Design review of the part shown in the three views and the two pictorial views. Dimensions are in mm from the part's minimum x, y and z. A direction names the side the tool comes from. Coordinates: 2 decimals unless noted, no trailing zeros. Loops run counter-clockwise (first coordinate to the right, second up) from the corner with the lowest first, then second, coordinate; pieces in that order, holes last. Notation, with made-up numbers: (22, -21) -> (78, -21) arc R20 ccw to (78, 16) -> close; hole circle Ø6 at (47.5, -15.5). An arc over 180 degrees is marked (long way). One line per item, written item: value. Start each with the question number.
1. Add section C-C on y = 33.5. Write out the cut boundary in (x, z), plus the area to 3 significant figures.
2. Add section A-A on y = 17.5. Write out the cut boundary in (x, z).
3. For probe 1 along X at (y, z) = (15, 6); probe 2 along Y at (x, z) = (80.2, 2.5); probe 3 along X at (y, z) = (46, 18.25), list the stretches that pass through material, from the lowest coordinate up.
4. Add section D-D on x = 16. Write out the cut boundary in (y, z).
5. Insertion check: pin 1 (2.5 mm diameter, centred on x = 80, z = 10, fed in from +Y); pin 2 (1.5 mm diameter, centred on x = 80.5, z = 1.5, fed in from -Y); pin 3 (4 mm diameter, centred on x = 72.5, z = 13.5, fed in from +Y). Each pin has a flat end and moves straight along its axis. Give the tip position at first contact, or say it passes through.
6. Machinability: for the marked faces 1, 2 and 3, which of the approach directions +Z, -Z, +X, -X, +Y, -Y give a long, thin tool a straight path to every point of the face, cutting with its end or side? Answer none if there is none.
7. Add section B-B on z = 2.5. Write out the cut boundary in (x, y).
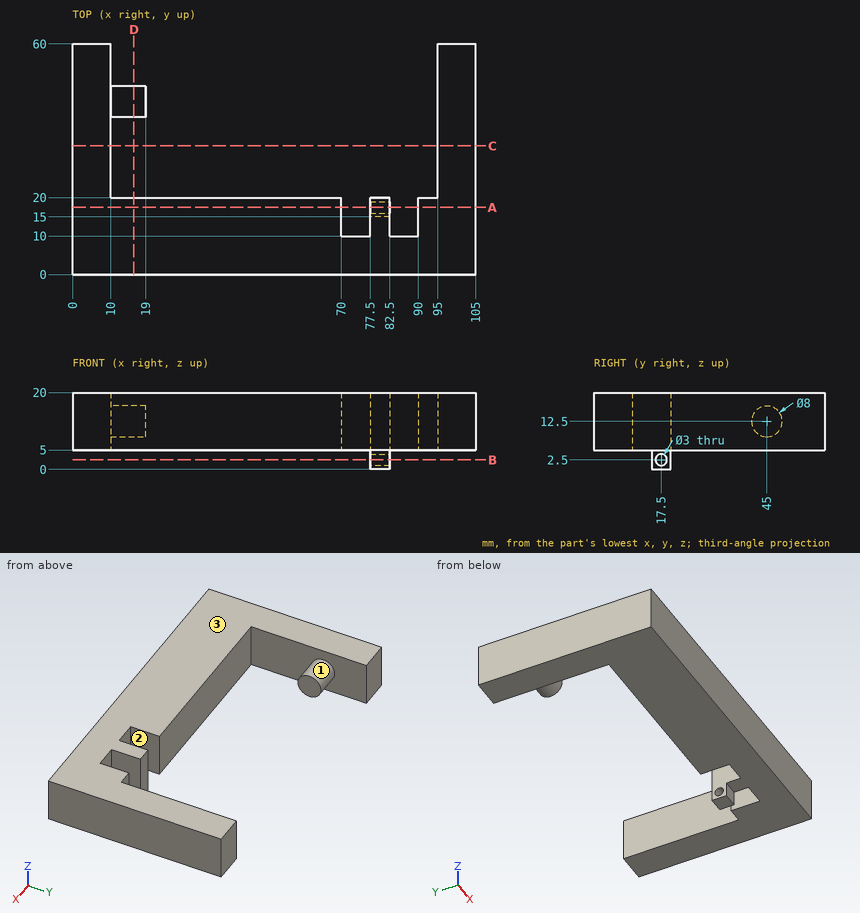
Worked answers:
1. outline: (0, 5) -> (10, 5) -> (10, 20) -> (0, 20) -> close; (95, 5) -> (105, 5) -> (105, 20) -> (95, 20) -> close
1. area: 300 mm²
2. outline: (0, 5) -> (70, 5) -> (70, 20) -> (0, 20) -> close; (77.5, 0) -> (82.5, 0) -> (82.5, 1) -> (77.5, 1) -> close; (77.5, 4) -> (82.5, 4) -> (82.5, 20) -> (77.5, 20) -> close; (90, 5) -> (105, 5) -> (105, 20) -> (90, 20) -> close
3. probe 1: x = 0 to 70, 77.5 to 82.5, 90 to 105
3. probe 2: y = 15 to 16, 19 to 20
3. probe 3: x = 0 to 10, 95 to 105
4. outline: (0, 5) -> (20, 5) -> (20, 20) -> (0, 20) -> close; circle Ø8 at (45, 12.5)
5. pin 1: stops at y = 20
5. pin 2: stops at y = 15
5. pin 3: stops at y = 10
6. face 1: none
6. face 2: +Z, -Z, +Y
6. face 3: +Z, +X, -X, +Y, -Y
7. outline: (77.5, 15) -> (82.5, 15) -> (82.5, 16) -> (77.5, 16) -> close; (77.5, 19) -> (82.5, 19) -> (82.5, 20) -> (77.5, 20) -> close
